Can you work these out from the model? Positions are in its coordinate system, mm. A direction names the side the tool comes from. Give positions to 0.01 mm unless a question says otherwise; leave off trailing zeros. Loops run counter-clockwise (first coordinate to the right, second up) from the corner with the lowest first, then second, coordinate; pieces in that order, holes last. Notation, with made-up numbers: M 85.5,79.5 L 89.5,79.5 A9 ccw 89.5,84.5 Z; hole C -5,5 d6. An arc over 180 degrees is marked long. Use CSV: the item, a comma, the result in double quotes.
Autodesk Inventor part; units mm, degrees
ref_plane "YZ Plane" through (0, 0, 0) normal (1, 0, 0) x (0, 1, 0)
ref_plane "XZ Plane" through (0, 0, 0) normal (0, 1, 0) x (-1, 0, 0)
ref_plane "XY Plane" through (0, 0, 0) normal (0, 0, 1) x (1, 0, 0)
sketch "Sketch9" plane through (0, 0, 0) normal (0, 0, 1) x (1, 0, 0)
  line L0 (1, 1) -> (1, -1)
  line L1 (1, -1) -> (-1, -1)
  line L2 (-1, -1) -> (-1, 1)
  line L3 (-1, 1) -> (1, 1)
  line L4 (-1.5, 1.5) -> (-1.5, -1.5)
  line L5 (-1.5, -1.5) -> (1.5, -1.5)
  line L6 (1.5, -1.5) -> (1.5, 1.5)
  line L7 (1.5, 1.5) -> (-1.5, 1.5)
  point P0 (0, 0)
  dimension "d36" = 2
  dimension "d37" = 3
extrude "Extrusion7" add sketch "Sketch9" along normal mid plane 6
sketch "Sketch10" plane through (0, 0, 0) normal (0, 0, 1) x (1, 0, 0)
  line L0 (-1.5, 1.5) -> (1.5, 1.5)
  line L1 (1.5, -1.5) -> (-1.5, -1.5)
  line L2 (0, 1.5) -> (0, -1.5) construction
  line L3 (0, 1.5) -> (-0.75, 1.5)
  line L4 (-0.75, 1.5) -> (-0.75, 2.5)
  line L5 (-0.75, 2.5) -> (0, 2.5)
  line L6 (0, 2.5) -> (0, 1.5)
  line L7 (0, -1.5) -> (-0.75, -1.5)
  line L8 (-0.75, -1.5) -> (-0.75, -2.5)
  line L9 (-0.75, -2.5) -> (0, -2.5)
  line L10 (0, -2.5) -> (0, -1.5)
  dimension "d40" = 0.75
  dimension "d42" = 1
  dimension "d43" = 1
revolve "Revolution2" add sketch "Sketch10" angle 360 about axis through (0, 1.5, 0) along (0, -1, 0)
properties part number "SlderA"
Q1. Please list where these lines run through material, in increasing order: L1, parallel to Y at x = 0.7, z = -0.8; L2, parallel to Y at x = 0.2, z = 0.45. Write a range as from..to.
Model answer:
L1,"-1.5..-1, 1..1.5"
L2,"-2.5..-1, 1..2.5"
Q2. I'm going to push a flat-ended pin straight in: P1, Ø1.5, axis at x = -0.5, z = -1.5, coming from the +Y side. Where does the tip first touch, or does it pass through?
Model answer:
P1,"y = 1.5"
Q3. I want a section at B-B, the plane z = 0. Please give me the cut outline in (x, y), then the cut area to 3 significant figures.
Model answer:
outline,"M -1.5,-1.5 L -0.75,-1.5 L -0.75,-2.5 L 0.75,-2.5 L 0.75,-1.5 L 1.5,-1.5 L 1.5,1.5 L 0.75,1.5 L 0.75,2.5 L -0.75,2.5 L -0.75,1.5 L -1.5,1.5 Z; hole M -1,-1 L 1,-1 L 1,1 L -1,1 Z"
area,"8.00 mm2"
Q4. I want a section at C-C, the plane x = -0.6. Please give me the cut outline in (y, z).
Model answer:
outline,"M -2.5,-0.45 L -1.5,-0.45 L -1.5,-3 L -1,-3 L -1,3 L -1.5,3 L -1.5,0.45 L -2.5,0.45 Z; M 1,-3 L 1.5,-3 L 1.5,-0.45 L 2.5,-0.45 L 2.5,0.45 L 1.5,0.45 L 1.5,3 L 1,3 Z"
Q5. For faces 1 (the flat face through (0, -1.5, -1)), 2 (the flat face through (0, 1.5, -1)), 3 (the flat face through (-1, 0, 0)), which set-ups out of +Z, -Z, +X, -X, +Y, -Y let a thin tool reach every point of the face, with its end or its side?
Model answer:
face 1,"-Y"
face 2,"+Y"
face 3,"+Z, -Z"
Q6. I want a section at D-D, the plane x = 0. Please give me the cut outline in (y, z), then the cut area to 3 significant figures.
Model answer:
outline,"M -2.5,-0.75 L -1.5,-0.75 L -1.5,-3 L -1,-3 L -1,3 L -1.5,3 L -1.5,0.75 L -2.5,0.75 Z; M 1,-3 L 1.5,-3 L 1.5,-0.75 L 2.5,-0.75 L 2.5,0.75 L 1.5,0.75 L 1.5,3 L 1,3 Z"
area,"9.00 mm2"
Q7. If we mould it in two halves opening along X, with no side actions, what happens to faces 4 (the cylindrical face through (0.75, -2.01, -0.03)), 5 (the flat face through (0, 1, 0)), 6 (the flat face through (-1.5, 0, 0))? For each: released by +X, released by -X, zero draft, split by the parting line, or undercut.
Model answer:
face 4,"split by the parting line"
face 5,"undercut"
face 6,"released by -X"
Q8. I want a section at A-A, the plane y = 0.15. Please give me the cut outline in (x, z).
Model answer:
outline,"M -1.5,-3 L -1,-3 L -1,3 L -1.5,3 Z; M 1,-3 L 1.5,-3 L 1.5,3 L 1,3 Z"
